The listing builds one solid part. Answer for the finished solid, in the listing's coordinates (mm). A direction names the side the tool comes from. Give positions to 0.01 mm unless a question says otherwise; leave off trailing zeros. Order: outer loops, then holes, each group sorted by start corner. A loop starts at its lowest first (then second) coordinate and runs counter-clockwise, first axis right, second up. Notation, with made-up numbers: (35.25, 1) - (89.25, 1) arc R24 cw to (89.25, 40) - close; hole circle Ø9 at (-10, 79.25). An arc over 180 degrees is marked (long way). Use a Markdown table: item, result. Add a question column.
1) The mould has two halves that part along Y. Classify faces 1 (the face through (30, -21, 0)), 2 (the face through (4.93, -15.43, 17)), 3 (the face through (55, 27, 0)): released by +Y, released by -Y, zero draft, split by the parting line, or undercut.
2) For faces 4 (the face through (4.93, 15.57, 17)), 5 (the face through (-10, 2, 0)), 6 (the face through (55, 24, -8)), 7 (the face through (30, 0, 21)), 8 (the face through (55, 24, 8)), determine the directions among +Z, -Z, +X, -X, +Y, -Y from which every point of the face is accessible in a straight line to the end or side of a thin tool.
3) Flat-ended cylindrical pins translate along their axes: pin 1 (1.8 mm diameter, centred on x = 56.5, y = 23.5, fed in from -Z); pin 2 (1.5 mm diameter, centred on y = -15, z = 15, fed in from -X); pin 3 (1.8 mm diameter, centred on x = 55, y = 23.5, fed in from +Z). Find the tip coordinate at first contact, or state that the pin passes through.
4) Straight lines are drawn through the part: line 1 (Y direction, x = 6, z = -15.5); line 2 (Z direction, x = 3, y = -15); line 3 (X direction, y = -2.5, z = -6.5). For each, find the intervals that lie inside material, in ascending order.
5) Find section D-D, the plane z = 0. Determine the outline of the cut face in (x, y).
6) Find section A-A, the plane z = -15.5. Determine the outline of the cut face in (x, y).
7) Find section C-C, the plane x = 53.5. Determine the outline of the cut face in (y, z).
from build123d import *

# Parameters (mm, degrees)
SKETCH_2_W          = 42
SKETCH_2_H          = 42
SKETCH_2_R          = 1.5
EXTRUDE_1_DEPTH     = 60
EXTRUDE_2_DEPTH     = 20
SKETCH_2_4_W        = 16
SKETCH_2_4_H        = 6
EXTRUDE_3_DEPTH     = 60
SKETCH_2_5_W        = 16
SKETCH_2_5_H        = 6
CUT_EXTRUDE_1_DEPTH = 51
SKETCH_2_6_R        = 1.5
EXTRUDE_4_DEPTH     = 60
SKETCH_2_7_R        = 1.5
CUT_EXTRUDE_2_DEPTH = 10


with BuildPart() as part:
    # Sketch 2 → Extrude 1 (new body)
    # profile 1 of 2: a face of its own
    with BuildSketch(Plane(origin=(0, 0, 0), x_dir=(0, 0, -1), z_dir=(1, 0, 0))):
        Rectangle(SKETCH_2_W, SKETCH_2_H)
        with Locations((15.5, -15.5)):
            Circle(SKETCH_2_R, mode=Mode.SUBTRACT)
        with Locations((15.5, 15.5)):
            Circle(SKETCH_2_R, mode=Mode.SUBTRACT)
        with Locations((-15.5, -15.5)):
            Circle(SKETCH_2_R, mode=Mode.SUBTRACT)
        with Locations((-15.5, 15.5)):
            Circle(SKETCH_2_R, mode=Mode.SUBTRACT)
        with BuildLine():
            ThreePointArc((-1.5, 2), (0, -2.5), (1.5, 2))
            Line((1.5, 2), (-1.5, 2))
        make_face(mode=Mode.SUBTRACT)
    # profile 2 of 2: a face of its own
    with BuildSketch(Plane(origin=(0, 0, 0), x_dir=(0, 0, -1), z_dir=(1, 0, 0))):
        with BuildLine():
            Line((-1.5, 2), (1.5, 2))
            ThreePointArc((1.5, 2), (0, -2.5), (-1.5, 2))
        make_face()
    extrude(amount=EXTRUDE_1_DEPTH)

    # Sketch 2_3 → Extrude 2 (add)
    with BuildSketch(Plane(origin=(0, 0, 0), x_dir=(0, 0, -1), z_dir=(1, 0, 0))):
        with BuildLine():
            Line((-1.5, 2), (1.5, 2))
            ThreePointArc((1.5, 2), (0, -2.5), (-1.5, 2))
        make_face()
    extrude(amount=-EXTRUDE_2_DEPTH)

    # Sketch 2_4 → Extrude 3 (add)
    with BuildSketch(Plane(origin=(0, 0, 0), x_dir=(0, 0, -1), z_dir=(1, 0, 0))):
        with Locations((0, 24)):
            Rectangle(SKETCH_2_4_W, SKETCH_2_4_H)
    extrude(amount=EXTRUDE_3_DEPTH)

    # Sketch 2_5 → Cut-Extrude 1 (cut)
    with BuildSketch(Plane(origin=(0, 0, 0), x_dir=(0, 0, -1), z_dir=(1, 0, 0))):
        with Locations((0, 24)):
            Rectangle(SKETCH_2_5_W, SKETCH_2_5_H)
    extrude(amount=CUT_EXTRUDE_1_DEPTH, mode=Mode.SUBTRACT)

    # Sketch 2_6 → Extrude 4 (add)
    with BuildSketch(Plane(origin=(0, 0, 0), x_dir=(0, 0, -1), z_dir=(1, 0, 0))):
        with Locations((15.5, 15.5)):
            Circle(SKETCH_2_6_R)
        with Locations((15.5, -15.5)):
            Circle(SKETCH_2_6_R)
        with Locations((-15.5, 15.5)):
            Circle(SKETCH_2_6_R)
        with Locations((-15.5, -15.5)):
            Circle(SKETCH_2_6_R)
    extrude(amount=EXTRUDE_4_DEPTH)

    # Sketch 2_7 → Cut-Extrude 2 (cut)
    with BuildSketch(Plane(origin=(0, 0, 0), x_dir=(0, 0, -1), z_dir=(1, 0, 0))):
        with Locations((-15.5, -15.5)):
            Circle(SKETCH_2_7_R)
        with Locations((-15.5, 15.5)):
            Circle(SKETCH_2_7_R)
        with Locations((15.5, 15.5)):
            Circle(SKETCH_2_7_R)
        with Locations((15.5, -15.5)):
            Circle(SKETCH_2_7_R)
    extrude(amount=CUT_EXTRUDE_2_DEPTH, mode=Mode.SUBTRACT)


solid = part.part
The answers:
| question | item | result |
|---|---|---|
| 1 | face 1 | released by -Y |
| 1 | face 2 | undercut |
| 1 | face 3 | released by +Y |
| 2 | face 4 | -X |
| 2 | face 5 | +Z, -Z, -X, +Y |
| 2 | face 6 | -Z, +X, -X, +Y |
| 2 | face 7 | +Z, +X, -X, +Y, -Y |
| 2 | face 8 | +Z, +X, -X, +Y |
| 3 | pin 1 | z = -8 |
| 3 | pin 2 | x = 10 |
| 3 | pin 3 | z = 8 |
| 4 | line 1 | -21 to -17, -14 to 14, 17 to 21 |
| 4 | line 2 | -21 to -16.91, -14.09 to 14.09, 16.91 to 21 |
| 4 | line 3 | 0 to 60 |
| 5 | outline | (-20, -2.5) - (0, -2.5) - (0, -21) - (60, -21) - (60, 27) - (51, 27) - (51, 21) - (0, 21) - (0, 2) - (-20, 2) - close |
| 6 | outline | (0, -21) - (60, -21) - (60, 21) - (0, 21) - (0, 17) - (10, 17) - (10, 14) - (0, 14) - (0, -14) - (10, -14) - (10, -17) - (0, -17) - close |
| 7 | outline | (-21, -21) - (21, -21) - (21, -8) - (27, -8) - (27, 8) - (21, 8) - (21, 21) - (-21, 21) - close |
